Autodesk Inventor part; units mm, degrees
ref_plane "YZ Plane" through (0, 0, 0) normal (1, 0, 0) x (0, 1, 0)
ref_plane "XZ Plane" through (0, 0, 0) normal (0, 1, 0) x (-1, 0, 0)
ref_plane "XY Plane" through (0, 0, 0) normal (0, 0, 1) x (1, 0, 0)
sketch "Sketch1" plane through (0, 0, 0) normal (0, 1, 0) x (-1, 0, 0)
  line L0 (-161.0144, 75.423) -> (-161.0144, -74.402)
  line L1 (-156.0144, 80.423) -> (179.5486, 80.423)
  arc A0 (-156.0144, 80.423) -> (-161.0144, 75.423) centre (-156.0144, 75.423) ccw
  arc A1 (-161.0144, -74.402) -> (-156.0144, -79.402) centre (-156.0144, -74.402) ccw
  line L2 (184.5486, -74.402) -> (184.5486, 75.423)
  line L3 (179.5486, -79.402) -> (-156.0144, -79.402)
  arc A2 (179.5486, -79.402) -> (184.5486, -74.402) centre (179.5486, -74.402) ccw
  arc A3 (184.5486, 75.423) -> (179.5486, 80.423) centre (179.5486, 75.423) ccw
  line L4 (-143.0264, 65.4235) -> (-72.3404, 65.4235)
  line L5 (169.5485, 62.4233) -> (169.5485, 33.0083)
  line L6 (-146.0144, -61.402) -> (-146.0144, -31.9917)
  line L7 (-146.0144, 62.4233) -> (-146.0144, 33.0083)
  line L8 (-156.0144, 0.5083) -> (-156.0144, -24.4917)
  line L9 (-156.0144, 0.5083) -> (-156.0144, 25.5083)
  line L10 (-151.0144, -29.4917) -> (-148.5144, -29.4917)
  line L11 (-151.0144, 30.5083) -> (-148.5144, 30.5083)
  line L12 (-7.3404, 65.4235) -> (30.8506, 65.4235)
  line L13 (166.5366, 65.4235) -> (95.8506, 65.4235)
  arc A4 (-151.0144, 30.5083) -> (-156.0144, 25.5083) centre (-151.0144, 25.5083) ccw
  arc A5 (-156.0144, -24.4917) -> (-151.0144, -29.4917) centre (-151.0144, -24.4917) ccw
  arc A6 (-146.0144, -31.9917) -> (-148.5144, -29.4917) centre (-148.5144, -31.9917) ccw
  arc A7 (-148.5144, 30.5083) -> (-146.0144, 33.0083) centre (-148.5144, 33.0083) ccw
  line L14 (179.5485, 0.5083) -> (179.5485, 25.5083)
  line L15 (179.5485, 0.5083) -> (179.5485, -24.4917)
  line L16 (174.5485, 30.5083) -> (172.0485, 30.5083)
  line L17 (174.5485, -29.4917) -> (172.0485, -29.4917)
  arc A8 (174.5485, -29.4917) -> (179.5485, -24.4917) centre (174.5485, -24.4917) ccw
  arc A9 (179.5485, 25.5083) -> (174.5485, 30.5083) centre (174.5485, 25.5083) ccw
  arc A10 (169.5485, 33.0083) -> (172.0485, 30.5083) centre (172.0485, 33.0083) ccw
  arc A11 (172.0485, -29.4917) -> (169.5485, -31.9917) centre (172.0485, -31.9917) ccw
  line L18 (169.5485, -31.9917) -> (169.5485, -61.402)
  line L19 (-39.8404, 75.4235) -> (-64.8404, 75.4235)
  line L20 (-39.8404, 75.4235) -> (-14.8404, 75.4235)
  line L21 (-69.8404, 70.4235) -> (-69.8404, 67.9235)
  line L22 (-9.8404, 70.4235) -> (-9.8404, 67.9235)
  arc A12 (-9.8404, 70.4235) -> (-14.8404, 75.4235) centre (-14.8404, 70.4235) ccw
  arc A13 (-64.8404, 75.4235) -> (-69.8404, 70.4235) centre (-64.8404, 70.4235) ccw
  arc A14 (-72.3404, 65.4235) -> (-69.8404, 67.9235) centre (-72.3404, 67.9235) ccw
  arc A15 (-9.8404, 67.9235) -> (-7.3404, 65.4235) centre (-7.3404, 67.9235) ccw
  line L23 (63.3506, 75.4235) -> (38.3506, 75.4235)
  line L24 (63.3506, 75.4235) -> (88.3506, 75.4235)
  line L25 (33.3506, 70.4235) -> (33.3506, 67.9235)
  line L26 (93.3506, 70.4235) -> (93.3506, 67.9235)
  arc A16 (93.3506, 70.4235) -> (88.3506, 75.4235) centre (88.3506, 70.4235) ccw
  arc A17 (38.3506, 75.4235) -> (33.3506, 70.4235) centre (38.3506, 70.4235) ccw
  arc A18 (30.8506, 65.4235) -> (33.3506, 67.9235) centre (30.8506, 67.9235) ccw
  arc A19 (93.3506, 67.9235) -> (95.8506, 65.4235) centre (95.8506, 67.9235) ccw
  line L27 (166.5485, -64.402) -> (95.8625, -64.402)
  line L28 (-143.0144, -64.402) -> (-72.3284, -64.402)
  line L29 (63.3625, -74.402) -> (88.3625, -74.402)
  line L30 (63.3625, -74.402) -> (38.3625, -74.402)
  line L31 (93.3625, -69.402) -> (93.3625, -66.902)
  line L32 (33.3625, -69.402) -> (33.3625, -66.902)
  arc A20 (33.3625, -69.402) -> (38.3625, -74.402) centre (38.3625, -69.402) ccw
  arc A21 (88.3625, -74.402) -> (93.3625, -69.402) centre (88.3625, -69.402) ccw
  arc A22 (95.8625, -64.402) -> (93.3625, -66.902) centre (95.8625, -66.902) ccw
  arc A23 (33.3625, -66.902) -> (30.8625, -64.402) centre (30.8625, -66.902) ccw
  line L33 (-39.8284, -74.402) -> (-14.8284, -74.402)
  line L34 (-39.8284, -74.402) -> (-64.8284, -74.402)
  line L35 (-9.8284, -69.402) -> (-9.8284, -66.902)
  line L36 (-69.8284, -69.402) -> (-69.8284, -66.902)
  arc A24 (-69.8284, -69.402) -> (-64.8284, -74.402) centre (-64.8284, -69.402) ccw
  arc A25 (-14.8284, -74.402) -> (-9.8284, -69.402) centre (-14.8284, -69.402) ccw
  arc A26 (-7.3284, -64.402) -> (-9.8284, -66.902) centre (-7.3284, -66.902) ccw
  arc A27 (-69.8284, -66.902) -> (-72.3284, -64.402) centre (-72.3284, -66.902) ccw
  line L37 (30.8625, -64.402) -> (-7.3284, -64.402)
  line L38 (-7.3284, -64.402) -> (11.7666, -64.402)
  line L39 (-7.3404, 65.4235) -> (11.7546, 65.4235)
  arc A28 (-143.0144, 65.4235) -> (-146.0144, 62.394) centre (-143.0144, 62.4233) ccw
  arc A29 (169.5485, 62.4233) -> (166.5366, 65.4235) centre (166.6427, 62.5181) ccw
  arc A30 (166.5485, -64.402) -> (169.5485, -61.402) centre (166.5485, -61.402) ccw
  arc A31 (-146.0144, -61.402) -> (-143.0144, -64.402) centre (-143.0144, -61.402) ccw
  point P0 (0, 0)
extrude "Extrusion1" add sketch "Sketch1" along normal blind 4
properties part number "layer3"
Can you work these out from the model? Positions are in its coordinate system, mm. Give positions to 0.01 mm unless a question says otherwise; leave off trailing zeros. Loops run counter-clockwise (first coordinate to the right, second up) from the corner with the lowest first, then second, coordinate; pieces in that order, holes last. Notation, with made-up numbers: (89.5, 36) - (104.5, 36) arc R23 ccw to (104.5, 69) - close; hole circle Ø4 at (-28.75, 31.25). An arc over 180 degrees is marked (long way). Return JSON: item names as keys, results as strings.
1. I want a section at A-A on z = 2. Please give me the cut outline in (x, y), and give its area (3 significant figures).
Output values:
{"outline": "(-184.55, 0) - (-179.55, 0) - (-179.55, 4) - (-184.55, 4) - close; (156.01, 0) - (161.01, 0) - (161.01, 4) - (156.01, 4) - close", "area": "40.0 mm²"}
2. If I drill on line 1 (X direction, y = 1.6, z = 68); line 2 (X direction, y = 0.35, z = 56); line 3 (Z direction, x = 108, y = 2.6), over which ranges is the centre line in solid material (lowest first)?
Output values:
{"line 1": "x = -184.55 to -93.35, -33.35 to 9.84, 69.84 to 161.01", "line 2": "x = -184.55 to -169.55, 146.01 to 161.01", "line 3": "z = -79.4 to -64.4, 65.42 to 80.42"}
3. I want a section at B-B on x = 50.5. Please give me the cut outline in (y, z), and give its area (3 significant figures).
Output values:
{"outline": "(0, -79.4) - (4, -79.4) - (4, -74.4) - (0, -74.4) - close; (0, 75.42) - (4, 75.42) - (4, 80.42) - (0, 80.42) - close", "area": "40.0 mm²"}
